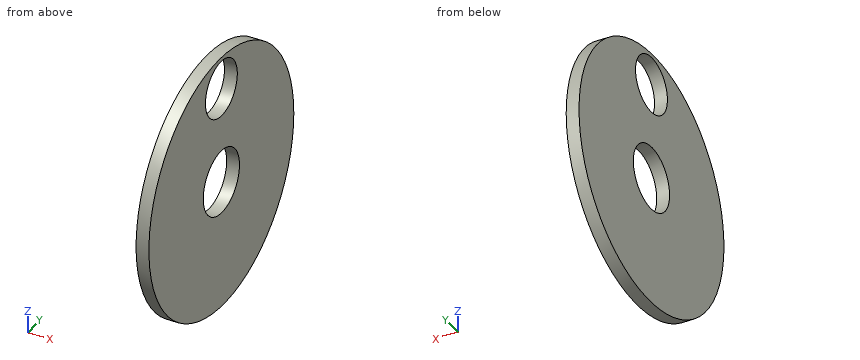
```python
from build123d import *

# Parameters (mm, degrees)
F0_R     = 50
F1_DEPTH = 2.5
F3_D     = 25
F5_D     = 22


with BuildPart() as f1:
    # F0 (on Right) → F1 (new body, symmetric)
    with BuildSketch(Plane.YZ):
        Circle(F0_R)
    extrude(amount=F1_DEPTH, both=True)

    # F3 (through all)
    with Locations(Plane.YZ.offset(2.5)):
        with Locations((0, 0)):
            Hole(F3_D / 2)

    # F5 (through all)
    with Locations(Plane.YZ.offset(2.5)):
        with Locations((0, 37.5)):
            Hole(F5_D / 2)


solid = f1.part
```
Build history of the part. All positions in model axes, mm. Round coordinates to 2 decimals unless told otherwise and drop trailing zeros. Loops run counter-clockwise (first coordinate to the right, second up) from the corner with the lowest first, then second, coordinate; pieces in that order, holes last.
Item 1: Saw through at C-C (x = 0.85). List the corners of the cut face in (y, z), then the cut area to 3 significant figures.
Item 2: Saw through at A-A (z = -4). List the corners of the cut face in (x, y).
Item 3: Saw through at D-D (z = 37.5). List the corners of the cut face in (x, y).
Item 4: Drill centre lines: line 1 along Z through (x, y) = (1.4, 0); line 2 along Z through (x, y) = (0.85, -7); line 3 along Y through (x, z) = (-1.3, 30.5). Where is each one in solid material? Low to high.
Item 5: Pin check, flat tips, straight feed: P1, Ø15, axis at y = 0, z = 0, coming from the +X side; P2, Ø1, axis at x = 0.5, y = 25.5, coming from the -Z side. Stop position of each tip, or through.
Item 6: Saw through at B-B (y = 0). List the corners of the cut face in (x, z).
Worked answers:
1. outline: circle Ø100 at (0, 0); hole circle Ø25 at (0, 0); hole circle Ø22 at (0, 37.5)
1. area: 6,980 mm2
2. outline: (-2.5, -49.84) - (2.5, -49.84) - (2.5, -11.84) - (-2.5, -11.84) - close; (-2.5, 11.84) - (2.5, 11.84) - (2.5, 49.84) - (-2.5, 49.84) - close
3. outline: (-2.5, -33.07) - (2.5, -33.07) - (2.5, -11) - (-2.5, -11) - close; (-2.5, 11) - (2.5, 11) - (2.5, 33.07) - (-2.5, 33.07) - close
4. line 1: z = -50 to -12.5, 12.5 to 26.5, 48.5 to 50
4. line 2: z = -49.51 to -10.36, 10.36 to 29.01, 45.99 to 49.51
4. line 3: y = -39.62 to -8.49, 8.49 to 39.62
5. P1: passes through
5. P2: stops at z = -43.3
6. outline: (-2.5, -50) - (2.5, -50) - (2.5, -12.5) - (-2.5, -12.5) - close; (-2.5, 12.5) - (2.5, 12.5) - (2.5, 26.5) - (-2.5, 26.5) - close; (-2.5, 48.5) - (2.5, 48.5) - (2.5, 50) - (-2.5, 50) - close
